The listing builds one solid part. Answer for the finished solid, in the listing's coordinates (mm). Face numbers are marked on the shaded views. A direction names the side the tool comes from. Coordinates: 2 decimals unless noted, no trailing zeros. Loops run counter-clockwise (first coordinate to the right, second up) from the corner with the lowest first, then second, coordinate; pieces in that order, holes last. Notation, with made-up numbers: M 84,23 L 121,23 A9 cw 121,40 Z; hole C -34,-34 d10. An arc over 180 degrees is marked long. Answer as a JSON object with one key per item and string values. Group by question number.
1. A cutting plane is placed at A-A on x = 0. Give the vertices of the cut face in (y, z).
2. For the marked faces 1 and 2, determine the directions among +Z, -Z, +X, -X, +Y, -Y from which every point of the face is accessible in a straight line to the end or side of a thin tool.
3. A cutting plane is placed at B-B on y = 36.5. Give the vertices of the cut face in (x, z), and give its area (3 significant figures).
4. A cutting plane is placed at C-C on z = 23. Give the vertices of the cut face in (x, y).
5. A cutting plane is placed at D-D on z = 0.5. Give the vertices of the cut face in (x, y).
6. Straight lines are drawn through the part: L1, parallel to Z at x = -22, y = -22; L2, parallel to Y at x = 2.5, z = 0; L3, parallel to Y at x = 10, z = 3. For each, find the intervals that lie inside material, in ascending order.
7. Given pin 1 (8 mm diameter, centred on y = -13, z = 13, fed in from +X); pin 2 (10 mm diameter, centred on x = -15, z = -0.5, fed in from +Y); pin 3 (8 mm diameter, centred on y = -25.5, z = 6.5, fed in from +X), each flat-ended and moving along its own axis, determine where each tip first touches the part or whether it passes through.
from build123d import *

# Parameters (mm, degrees)
F0_R     = 46.318814
F1_DEPTH = 5
F2_R     = 5
F3_DEPTH = 25


with BuildPart() as f1:
    # F0 (on Top) → F1 (new body, symmetric)
    with BuildSketch(Plane.XY):
        Circle(F0_R)
    extrude(amount=F1_DEPTH, both=True)

    # F2 (on face) → F3 (join)
    with BuildSketch(Plane.XY.offset(5)):
        with Locations((0, 35)):
            Circle(F2_R)
        with Locations((-30.310889, -17.5)):
            Circle(F2_R)
        with Locations((30.310889, -17.5)):
            Circle(F2_R)
    extrude(amount=F3_DEPTH)


solid = f1.part
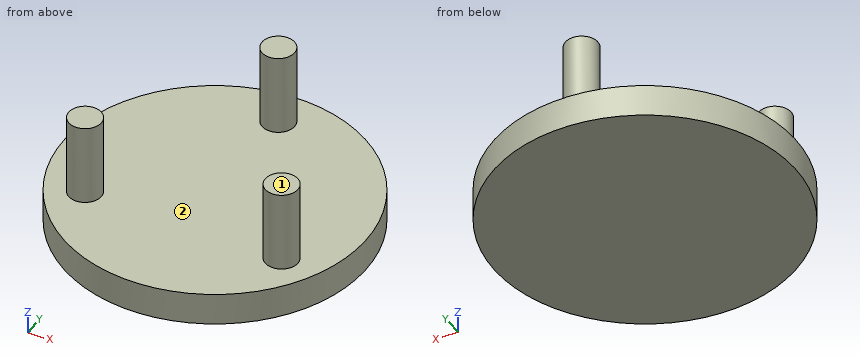
From the geometry:
{
 "1": {"outline": "M -46.32,-5 L 46.32,-5 L 46.32,5 L 40,5 L 40,30 L 30,30 L 30,5 L -46.32,5 Z"},
 "2": {"face 1": "+Z, +X, -X, +Y, -Y", "face 2": "+Z"},
 "3": {"outline": "M -28.52,-5 L 28.52,-5 L 28.52,5 L 4.77,5 L 4.77,30 L -4.77,30 L -4.77,5 L -28.52,5 Z", "area": "809 mm²"},
 "4": {"outline": "C -30.31,-17.5 d10; C 0,35 d10; C 30.31,-17.5 d10"},
 "5": {"outline": "C 0,0 d92.64"},
 "6": {"L1": "z = -5 to 5", "L2": "y = -46.25 to 46.25", "L3": "y = -45.23 to 45.23"},
 "7": {"pin 1": "stops at x = 35.29", "pin 2": "stops at y = 45.23", "pin 3": "stops at x = 40.87"}
}
